Geometry: final body of the model. Coordinates: model frame, mm. Round coordinates to 2 decimals unless told otherwise and drop trailing zeros. Loops run counter-clockwise (first coordinate to the right, second up) from the corner with the lowest first, then second, coordinate; pieces in that order, holes last. Notation, with made-up numbers: M 64,52 L 101,52 A15 ccw 101,76 Z; hole C 69.5,-39.5 d4. An arc over 180 degrees is marked long. Write each question's results on one line, items separated by ' | '.
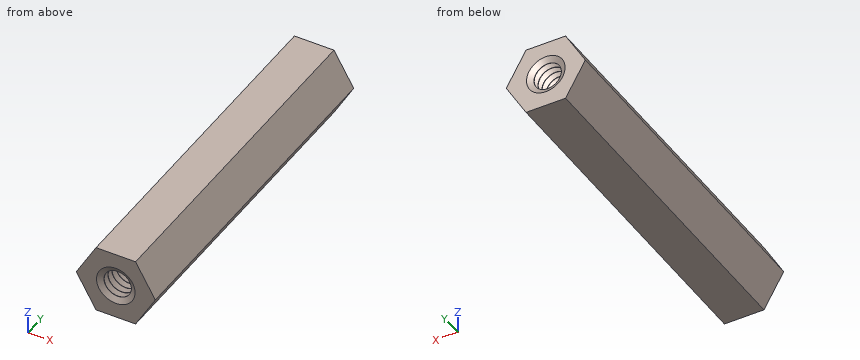
```python
from build123d import *

# Parameters (mm, degrees)
BOSS_EXTRUDE1_DEPTH = 10
SKETCH3_R           = 0.8
CUT_EXTRUDE1_DEPTH  = 20
LPATTERN3_COUNT     = 15
LPATTERN3_PITCH     = 0.4


with BuildPart() as part:
    # Sketch1 → Boss-Extrude1 (new body, symmetric)
    with BuildSketch(Plane(origin=(0, 0, 0), x_dir=(1, 0, 0), z_dir=(0, 1, 0))):
        Polygon((2.309401077, 0), (1.154700538, 2), (-1.154700538, 2), (-2.309401077, 0), (-1.154700538, -2), (1.154700538, -2), align=None)
    extrude(amount=BOSS_EXTRUDE1_DEPTH, both=True)

    # Sketch3 → Cut-Extrude1 (cut)
    with BuildSketch(Plane.XZ.offset(10)):
        Circle(SKETCH3_R)
    extrude(amount=-CUT_EXTRUDE1_DEPTH, mode=Mode.SUBTRACT)

    # Sketch5 → Cut-Revolve3 (revolve, cut)
    with BuildSketch(Plane.XY):
        Polygon((0.38, -9.8), (0.38, -10.2), (0.78, -10.2), (1.126410162, -10), (0.78, -9.8), align=None)
    cut_revolve3 = revolve(axis=Axis((0, 0, 0), (0, -1, 0)), mode=Mode.SUBTRACT)

    # LPattern3: Cut-Revolve3 ×15
    with Locations(*[(0, i * LPATTERN3_PITCH, 0) for i in range(1, LPATTERN3_COUNT)]):
        add(cut_revolve3, mode=Mode.SUBTRACT)

    # Mirror2: Cut-Revolve3 across plane
    add(cut_revolve3.mirror(Plane.ZX), mode=Mode.SUBTRACT)

    # Mirror2 copy 1 sketch → Mirror2 copy 1 (revolve, cut)
    with BuildSketch(Plane(origin=(0, -0.4, 0), x_dir=(1, 0, 0), z_dir=(0, 0, 1))):
        Polygon((0.38, 9.8), (0.38, 10.2), (0.78, 10.2), (1.126410162, 10), (0.78, 9.8), align=None)
    revolve(axis=Axis((0, -0.4, 0), (0, -1, 0)), mode=Mode.SUBTRACT)

    # Mirror2 copy 2 sketch → Mirror2 copy 2 (revolve, cut)
    with BuildSketch(Plane(origin=(0, -0.8, 0), x_dir=(1, 0, 0), z_dir=(0, 0, 1))):
        Polygon((0.38, 9.8), (0.38, 10.2), (0.78, 10.2), (1.126410162, 10), (0.78, 9.8), align=None)
    revolve(axis=Axis((0, -0.8, 0), (0, -1, 0)), mode=Mode.SUBTRACT)

    # Mirror2 copy 3 sketch → Mirror2 copy 3 (revolve, cut)
    with BuildSketch(Plane(origin=(0, -1.2, 0), x_dir=(1, 0, 0), z_dir=(0, 0, 1))):
        Polygon((0.38, 9.8), (0.38, 10.2), (0.78, 10.2), (1.126410162, 10), (0.78, 9.8), align=None)
    revolve(axis=Axis((0, -1.2, 0), (0, -1, 0)), mode=Mode.SUBTRACT)

    # Mirror2 copy 4 sketch → Mirror2 copy 4 (revolve, cut)
    with BuildSketch(Plane(origin=(0, -1.6, 0), x_dir=(1, 0, 0), z_dir=(0, 0, 1))):
        Polygon((0.38, 9.8), (0.38, 10.2), (0.78, 10.2), (1.126410162, 10), (0.78, 9.8), align=None)
    revolve(axis=Axis((0, -1.6, 0), (0, -1, 0)), mode=Mode.SUBTRACT)

    # Mirror2 copy 5 sketch → Mirror2 copy 5 (revolve, cut)
    with BuildSketch(Plane(origin=(0, -2, 0), x_dir=(1, 0, 0), z_dir=(0, 0, 1))):
        Polygon((0.38, 9.8), (0.38, 10.2), (0.78, 10.2), (1.126410162, 10), (0.78, 9.8), align=None)
    revolve(axis=Axis((0, -2, 0), (0, -1, 0)), mode=Mode.SUBTRACT)

    # Mirror2 copy 6 sketch → Mirror2 copy 6 (revolve, cut)
    with BuildSketch(Plane(origin=(0, -2.4, 0), x_dir=(1, 0, 0), z_dir=(0, 0, 1))):
        Polygon((0.38, 9.8), (0.38, 10.2), (0.78, 10.2), (1.126410162, 10), (0.78, 9.8), align=None)
    revolve(axis=Axis((0, -2.4, 0), (0, -1, 0)), mode=Mode.SUBTRACT)

    # Mirror2 copy 7 sketch → Mirror2 copy 7 (revolve, cut)
    with BuildSketch(Plane(origin=(0, -2.8, 0), x_dir=(1, 0, 0), z_dir=(0, 0, 1))):
        Polygon((0.38, 9.8), (0.38, 10.2), (0.78, 10.2), (1.126410162, 10), (0.78, 9.8), align=None)
    revolve(axis=Axis((0, -2.8, 0), (0, -1, 0)), mode=Mode.SUBTRACT)

    # Mirror2 copy 8 sketch → Mirror2 copy 8 (revolve, cut)
    with BuildSketch(Plane(origin=(0, -3.2, 0), x_dir=(1, 0, 0), z_dir=(0, 0, 1))):
        Polygon((0.38, 9.8), (0.38, 10.2), (0.78, 10.2), (1.126410162, 10), (0.78, 9.8), align=None)
    revolve(axis=Axis((0, -3.2, 0), (0, -1, 0)), mode=Mode.SUBTRACT)

    # Mirror2 copy 9 sketch → Mirror2 copy 9 (revolve, cut)
    with BuildSketch(Plane(origin=(0, -3.6, 0), x_dir=(1, 0, 0), z_dir=(0, 0, 1))):
        Polygon((0.38, 9.8), (0.38, 10.2), (0.78, 10.2), (1.126410162, 10), (0.78, 9.8), align=None)
    revolve(axis=Axis((0, -3.6, 0), (0, -1, 0)), mode=Mode.SUBTRACT)

    # Mirror2 copy 10 sketch → Mirror2 copy 10 (revolve, cut)
    with BuildSketch(Plane(origin=(0, -4, 0), x_dir=(1, 0, 0), z_dir=(0, 0, 1))):
        Polygon((0.38, 9.8), (0.38, 10.2), (0.78, 10.2), (1.126410162, 10), (0.78, 9.8), align=None)
    revolve(axis=Axis((0, -4, 0), (0, -1, 0)), mode=Mode.SUBTRACT)

    # Mirror2 copy 11 sketch → Mirror2 copy 11 (revolve, cut)
    with BuildSketch(Plane(origin=(0, -4.4, 0), x_dir=(1, 0, 0), z_dir=(0, 0, 1))):
        Polygon((0.38, 9.8), (0.38, 10.2), (0.78, 10.2), (1.126410162, 10), (0.78, 9.8), align=None)
    revolve(axis=Axis((0, -4.4, 0), (0, -1, 0)), mode=Mode.SUBTRACT)

    # Mirror2 copy 12 sketch → Mirror2 copy 12 (revolve, cut)
    with BuildSketch(Plane(origin=(0, -4.8, 0), x_dir=(1, 0, 0), z_dir=(0, 0, 1))):
        Polygon((0.38, 9.8), (0.38, 10.2), (0.78, 10.2), (1.126410162, 10), (0.78, 9.8), align=None)
    revolve(axis=Axis((0, -4.8, 0), (0, -1, 0)), mode=Mode.SUBTRACT)

    # Mirror2 copy 13 sketch → Mirror2 copy 13 (revolve, cut)
    with BuildSketch(Plane(origin=(0, -5.2, 0), x_dir=(1, 0, 0), z_dir=(0, 0, 1))):
        Polygon((0.38, 9.8), (0.38, 10.2), (0.78, 10.2), (1.126410162, 10), (0.78, 9.8), align=None)
    revolve(axis=Axis((0, -5.2, 0), (0, -1, 0)), mode=Mode.SUBTRACT)

    # Mirror2 copy 14 sketch → Mirror2 copy 14 (revolve, cut)
    with BuildSketch(Plane(origin=(0, -5.6, 0), x_dir=(1, 0, 0), z_dir=(0, 0, 1))):
        Polygon((0.38, 9.8), (0.38, 10.2), (0.78, 10.2), (1.126410162, 10), (0.78, 9.8), align=None)
    revolve(axis=Axis((0, -5.6, 0), (0, -1, 0)), mode=Mode.SUBTRACT)


solid = part.part
```
1. Pin query (flat end, axial travel): P1, Ø1.5, axis at y = -8, z = 1, coming from the +X side; P2, Ø1, axis at y = 4.5, z = -1.5, coming from the -X side; P3, Ø2, axis at x = 0, z = 0, coming from the +Y side. Return the tip coordinate at first contact, or that it passes through.
Answer key:
P1: stops at x = 2.17 | P2: stops at x = -1.73 | P3: stops at y = 9.93
2. Section A-A (y = -1). Output: boundary loops of the cut face in (x, z), then the cut area to 3 significant figures.
Answer key:
outline: M -2.31,0 L -1.15,-2 L 1.15,-2 L 2.31,0 L 1.15,2 L -1.15,2 Z; hole C 0,0 d1.6 | area: 11.8 mm²
3. Section C-C (z = 1.3). Output: boundary loops of the cut face in (x, y).
Answer key:
outline: M -1.56,-10 L 1.56,-10 L 1.56,10 L -1.56,10 Z
4. Section B-B (x = -1.9). Output: boundary loops of the cut face in (y, z).
Answer key:
outline: M -10,-0.71 L 10,-0.71 L 10,0.71 L -10,0.71 Z
5. Ray query, probe 1 along Z at (x, y) = (-0.3, 2.5); probe 2 along X at (y, z) = (7.25, 0.25); probe 3 along Z at (x, y) = (0, 9.05). Return the intervals inside material, ascending.
Answer key:
probe 1: z = -2 to -0.74, 0.74 to 2 | probe 2: x = -2.17 to -1.01, 1.01 to 2.17 | probe 3: z = -2 to -0.87, 0.87 to 2
